Source: CAD feature listing. Evaluate the final solid. Frame: model axes, mm. A direction names the side the tool comes from. Coordinates: 2 decimals unless noted, no trailing zeros. Write each loop counter-clockwise with the first axis right and the second up, starting at its lowest first coordinate (ties: lowest second). Pieces come first, ordered by that corner, then holes. Notation, with made-up numbers: (13.25, -21) -> (69.25, -21) arc R33 cw to (69.25, 12) -> close; hole circle Ø10 at (-13, 31). An arc over 180 degrees is marked (long way). Write item = value, one per line.
from build123d import *

# Parameters (mm, degrees)
F0_R      = 25
F0_R_2    = 20
F1_DEPTH  = 500
F2_R      = 25
F3_DEPTH  = 5
F5_DEPTH  = 20
F7_D      = 5
F10_D     = 12
F10_DEPTH = 6
F10_START = 0.7306779
F10_TIP   = 3.6051637142
F12_DEPTH = 20
F17_D     = 12
F17_DEPTH = 6
F17_START = 0.7306779
F17_TIP   = 3.6051637142
F19_D     = 12
F19_DEPTH = 6
F19_START = 0.7306779
F19_TIP   = 3.6051637142


with BuildPart() as f1:
    # F0 (on Front) → F1 (new body)
    with BuildSketch(Plane.XZ):
        Circle(F0_R)
        Circle(F0_R_2, mode=Mode.SUBTRACT)
    extrude(amount=F1_DEPTH)

    # F2 (on face) → F3 (join)
    with BuildSketch(Plane.XZ.offset(500)):
        Circle(F2_R)
    extrude(amount=F3_DEPTH)

    # F4 (on face) → F5 (join)
    with BuildSketch(Plane.XZ.offset(505)):
        Polygon((-16.0628025015, -5.6190539991), (0.380358971, -17.013016167), (16.2978772735, -4.8955682433), (9.6922831285, 13.9873885984), (-10.3077168715, 13.540249811), align=None)
    extrude(amount=F5_DEPTH)

    # F7 (through all)
    with Locations(Plane.XZ.offset(525)):
        with Locations((0, 0)):
            Hole(F7_D / 2)

    # F10
    # its depths count from where the whole tool has entered the part; down to there all is cleared
    with Locations(Plane.YZ.offset(25).offset(-F10_START)):
        with Locations((-20, 0), (-130, 0)):
            Hole(F10_D / 2, depth=F10_DEPTH)
            with Locations((0, 0, -(F10_DEPTH + F10_TIP / 2))):  # 118° drill point
                Cone(0, F10_D / 2, F10_TIP, mode=Mode.SUBTRACT)

    # F11 (on face) → F12 (join)
    with BuildSketch(Plane(origin=(0, 0, 0), x_dir=(-1, 0, 0), z_dir=(0, 1, 0))):
        Polygon((12.5, -21.6506350946), (12.5, 21.6506350946), (-25, 0), align=None)
    extrude(amount=F12_DEPTH)

    # F17
    # its depths count from where the whole tool has entered the part; down to there all is cleared
    with Locations(Plane(origin=(-12.5, 0, -21.6506350946), x_dir=(0.8660254038, 0, -0.5), z_dir=(-0.5, 0, -0.8660254038)).offset(-F17_START)):
        with Locations((0, 20), (0, 130)):
            Hole(F17_D / 2, depth=F17_DEPTH)
            with Locations((0, 0, -(F17_DEPTH + F17_TIP / 2))):  # 118° drill point
                Cone(0, F17_D / 2, F17_TIP, mode=Mode.SUBTRACT)

    # F19
    # its depths count from where the whole tool has entered the part; down to there all is cleared
    with Locations(Plane(origin=(-12.5, 0, 21.6506350946), x_dir=(0.8660254038, 0, 0.5), z_dir=(-0.5, 0, 0.8660254038)).offset(-F19_START)):
        with Locations((0, -20), (0, -130)):
            Hole(F19_D / 2, depth=F19_DEPTH)
            with Locations((0, 0, -(F19_DEPTH + F19_TIP / 2))):  # 118° drill point
                Cone(0, F19_D / 2, F19_TIP, mode=Mode.SUBTRACT)


solid = f1.part
1) Cut plane B-B, the plane y = -297. Output: boundary loops of the cut face in (x, z), and give its area (3 significant figures).
Answer block:
outline = circle Ø50 at (0, 0); hole circle Ø40 at (0, 0)
area = 707 mm2
2) First-contact query: pin 1 Ø6 at (x, z) = (16.5, 13.5) entering from -Y; pin 2 Ø6 at (x, y) = (4, -202) entering from +Z; pin 3 Ø6 at (y, z) = (11, 5.5) entering from -X. Flat tips, straight axial feed; report the tip coordinate or a pass-through.
Answer block:
pin_1 = -505
pin_2 = 24.98
pin_3 = -12.5
3) Pull-direction query (Y, two-part tool) for faces 4 (the flat face through (-13.145, -514.86, 4.095)), 5 (the flat face through (-20.2, 0, 0.3)), 6 (the cylindrical face through (-15.954, -131.802, -16.187)), 7 (the flat face through (3, -525, -1)); classes: +Y half, -Y half, draft (parallel to the pull), parting line (faces both ways), or undercut.
Answer block:
face_4 = draft
face_5 = +Y half
face_6 = undercut
face_7 = -Y half
4) Reachability of faces 1 (the flat face through (13.041, -514.86, 4.414)), 2 (the flat face through (-12.5, 10, 0)), 3 (the cylindrical face through (22, -25.54, -2.3)) from +Z, -Z, +X, -X, +Y, -Y: full face, straight path, thin tool, end or side. Return the list, or none.
Answer block:
face_1 = +Z, +X, -Y
face_2 = +Z, -Z, -X, +Y
face_3 = +X
5) Material intervals for probe 1 along Y at (x, z) = (-11, 19); probe 2 along Y at (x, z) = (8, 7.5); probe 3 along Z at (x, y) = (0, -400), sorted ascending. Write a range as [from, to].
Answer block:
probe_1 = [-505, -136], [-124, -26], [-14, 20]
probe_2 = [-525, -500], [0, 20]
probe_3 = [-25, -20], [20, 25]
6) Cut plane A-A, the plane y = -130. Output: boundary loops of the cut face in (x, z).
Answer block:
outline = (-17.33, -18.02) -> (-14.74, -13.52) arc R20 cw to (-14.74, 13.52) -> (-17.33, 18.02) arc R25 ccw to start; (-6.94, -24.02) arc R25 ccw to (24.27, -6) -> (19.08, -6) arc R20 cw to (-4.34, -19.52) -> close; (-6.94, 24.02) -> (-4.34, 19.52) arc R20 cw to (19.08, 6) -> (24.27, 6) arc R25 ccw to start
